Model file for the job. Use its own axes, mm. Face numbers are marked on the shaded views. A direction names the side the tool comes from. Give positions to 0.01 mm unless a question says otherwise; leave off trailing zeros. Answer in a Markdown table with one row per item.
```python
from build123d import *

# Parameters (mm, degrees)
SKETCH1_R                = 34.544
BOSS_EXTRUDE1_DEPTH      = 7.62
SKETCH2_R                = 28.1686
CUT_EXTRUDE1_DEPTH       = 3.048
CUT_EXTRUDE2_START       = -1.778
SKETCH3_R                = 28.1686
SKETCH3_R_2              = 4.3688
CUT_EXTRUDE2_DEPTH       = 1.778
CUT_EXTRUDE3_DEPTH       = 50.200658898
FILLET1_R                = 1.6002
CIRPATTERN1_COUNT        = 5
FILLET1_OF_CIRPATTERN1_R = 1.6002
SKETCH5_R                = 17.4625
SKETCH5_R_2              = 10.7061
BOSS_EXTRUDE2_DEPTH      = 1.778
BOSS_EXTRUDE4_START      = 1.6002
SKETCH6_R                = 17.4625
SKETCH6_R_2              = 16.4211
BOSS_EXTRUDE4_DEPTH      = 1.6002
SKETCH7_R                = 3.175
CUT_EXTRUDE4_DEPTH       = 50.066068275
SKETCH8_R                = 1.4224
CUT_EXTRUDE5_DEPTH       = 50.066068275
CIRPATTERN2_COUNT        = 5
BOSS_EXTRUDE5_DEPTH      = 0.0254
BOSS_EXTRUDE5_DEPTH_BACK = 7.6454
SKETCH9_R                = 34.5567
SKETCH9_R_2              = 30.4165


with BuildPart() as part:
    # Sketch1 → Boss-Extrude1 (new body)
    with BuildSketch(Plane(origin=(0, 0, 0), x_dir=(0, 0, -1), z_dir=(1, 0, 0))):
        with Locations(Location((0, 0, 0), (0, 0, 180))):
            Circle(SKETCH1_R)
    extrude(amount=BOSS_EXTRUDE1_DEPTH)

    # Sketch2 → Cut-Extrude1 (cut)
    with BuildSketch(Plane(origin=(7.62, 0, 0), x_dir=(0, 0, -1), z_dir=(1, 0, 0))):
        Circle(SKETCH2_R)
    extrude(amount=-CUT_EXTRUDE1_DEPTH, mode=Mode.SUBTRACT)

    # Sketch3 → Cut-Extrude2 (cut)
    with BuildSketch(Plane.ZY.offset(CUT_EXTRUDE2_START)):
        with Locations(Location((0, 0, 0), (0, 0, 180))):
            Circle(SKETCH3_R)
        Circle(SKETCH3_R_2, mode=Mode.SUBTRACT)
    extrude(amount=CUT_EXTRUDE2_DEPTH, mode=Mode.SUBTRACT)

    # Sketch4 → Cut-Extrude3 (cut, through all)
    with BuildSketch(Plane.ZY.offset(-1.778)):
        with BuildLine():
            Line((-2.54, 6.985), (2.54, 6.985))
            Line((2.54, 6.985), (9.114287493, 25.064290604))
            ThreePointArc((9.114287493, 25.064290604), (0, 26.67), (-9.114287493, 25.064290604))
            Line((-9.114287493, 25.064290604), (-2.54, 6.985))
        make_face()
    cut_extrude3 = extrude(amount=-CUT_EXTRUDE3_DEPTH, mode=Mode.SUBTRACT)

    # Fillet1
    fillet1_edges = [part.edges().sort_by_distance(p)[0] for p in [
        (3.175, 25.064290604, 9.114287493),
        (3.175, 6.985, 2.54),
        (3.175, 6.985, -2.54),
        (3.175, 25.064290604, -9.114287493),
    ]]
    fillet(fillet1_edges, radius=FILLET1_R)

    # CirPattern1: Cut-Extrude3 ×5 about axis
    cirpattern1_axis = Axis((0, 0, 0), (1, 0, 0))
    for i in range(1, CIRPATTERN1_COUNT):
        add(cut_extrude3.rotate(cirpattern1_axis, i * 360 / CIRPATTERN1_COUNT), mode=Mode.SUBTRACT)

    # Fillet1 of CirPattern1
    fillet1_of_cirpattern1_edges = [part.edges().sort_by_distance(p)[0] for p in [
        (3.175, -0.922910762, 26.654026632),
        (3.175, -0.257199846, 7.428032932),
        (3.175, 4.574167257, 5.858226601),
        (3.175, 16.41349426, 21.021087179),
        (3.175, -25.634680824, 7.358806903),
        (3.175, -7.143958247, 2.050776822),
        (3.175, -4.158009165, 6.160583153),
        (3.175, -14.920193278, 22.10603385),
        (3.175, -14.920193278, -22.10603385),
        (3.175, -4.158009165, -6.160583153),
        (3.175, -7.143958247, -2.050776822),
        (3.175, -25.634680824, -7.358806903),
        (3.175, 16.41349426, -21.021087179),
        (3.175, 4.574167257, -5.858226601),
        (3.175, -0.257199846, -7.428032932),
        (3.175, -0.922910762, -26.654026632),
    ]]
    fillet(fillet1_of_cirpattern1_edges, radius=FILLET1_OF_CIRPATTERN1_R)

    # Sketch5 → Boss-Extrude2 (add)
    with BuildSketch(Plane(origin=(4.572, 0, 0), x_dir=(0, 0, -1), z_dir=(1, 0, 0))):
        Circle(SKETCH5_R)
        Circle(SKETCH5_R_2, mode=Mode.SUBTRACT)
    extrude(amount=-BOSS_EXTRUDE2_DEPTH)

    # Sketch6 → Boss-Extrude4 (add)
    with BuildSketch(Plane(origin=(4.572, 0, 0), x_dir=(0, 0, -1), z_dir=(1, 0, 0)).offset(BOSS_EXTRUDE4_START)):
        Circle(SKETCH6_R)
        Circle(SKETCH6_R_2, mode=Mode.SUBTRACT)
    extrude(amount=-BOSS_EXTRUDE4_DEPTH)

    # Sketch7 → Cut-Extrude4 (cut, through all)
    with BuildSketch(Plane(origin=(4.572, 0, 0), x_dir=(0, 0, -1), z_dir=(1, 0, 0))):
        Circle(SKETCH7_R)
    extrude(amount=-CUT_EXTRUDE4_DEPTH, mode=Mode.SUBTRACT)

    # Sketch8 → Cut-Extrude5 (cut, through all)
    with BuildSketch(Plane(origin=(4.572, 0, 0), x_dir=(0, 0, -1), z_dir=(1, 0, 0))):
        with Locations((0, -6.35)):
            Circle(SKETCH8_R)
    cut_extrude5 = extrude(amount=-CUT_EXTRUDE5_DEPTH, mode=Mode.SUBTRACT)

    # CirPattern2: Cut-Extrude5 ×5 about axis
    cirpattern2_axis = Axis((0, 0, 0), (1, 0, 0))
    for i in range(1, CIRPATTERN2_COUNT):
        add(cut_extrude5.rotate(cirpattern2_axis, i * 360 / CIRPATTERN2_COUNT), mode=Mode.SUBTRACT)

    # Sketch9 → Boss-Extrude5 (add, two sides: drawn at the far end of the back side and taken through both)
    with BuildSketch(Plane(origin=(7.62, 0, 0), x_dir=(0, 0, -1), z_dir=(1, 0, 0)).offset(-BOSS_EXTRUDE5_DEPTH_BACK)):
        Circle(SKETCH9_R)
        Circle(SKETCH9_R_2, mode=Mode.SUBTRACT)
    extrude(amount=BOSS_EXTRUDE5_DEPTH + BOSS_EXTRUDE5_DEPTH_BACK)


solid = part.part
```
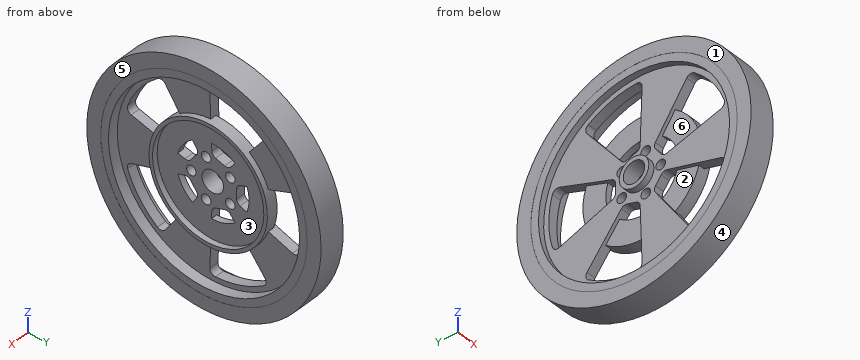
(1) Saw through at A-A, the plane y = -15. Count the separate pieces of the cut face and the enclosed holes in it, and give its area (3 significant figures).
Established:
| item | result |
|---|---|
| separate pieces | 3 |
| enclosed holes | 0 |
| area | 173 mm2 |
(2) Wall check: L1, parallel to Y at x = 0.4, z = 0 (3 decimals); L2, parallel to Y at x = 5.3, z = 0; L3, parallel to Z at x = 5.5, y = -10. Give the ranges that are in metal, low to high.
Established:
| item | result |
|---|---|
| L1 | y = -34.557 to -28.169, -4.369 to -3.175, 3.175 to 4.369, 28.169 to 34.557 |
| L2 | y = -34.56 to -28.17, -17.46 to -16.42, 16.42 to 17.46, 28.17 to 34.56 |
| L3 | z = -33.08 to -26.33, -14.32 to -13.03, 13.03 to 14.32, 26.33 to 33.08 |
(3) Flat gauge pins, fed straight in: P1, Ø10, axis at y = 0, z = 3.5, coming from the +X side; P2, Ø4.5, axis at y = 7, z = -12, coming from the -X side; P3, Ø2, axis at x = 1.5, y = 18, coming from the -Z side; P4, Ø2.5, axis at y = -6.35, z = 0, coming from the -X side. Where does each tip first touch, or does it go through?
Established:
| item | result |
|---|---|
| P1 | stops at x = 4.57 |
| P2 | stops at x = 1.78 |
| P3 | stops at z = -30.09 |
| P4 | passes through |
(4) Mould opens along Z. For the marked faces 4, 5 and 6 say: pulls with the +Z half, pulls with the -Z half, needs draft (parallel to the pull), parting line crosses it, or undercut.
Established:
| item | result |
|---|---|
| face 4 | parting line crosses it |
| face 5 | needs draft |
| face 6 | undercut |
(5) Which spindle directions (+Z, -Z, +X, -X, +Y, -Y) get a long thin tool onto all of the face, cutting with end or side? Do the marked faces 1, 2 and 3. Say none if no direction does.
Established:
| item | result |
|---|---|
| face 1 | +Z, -Z, -X, +Y, -Y |
| face 2 | -X |
| face 3 | +X |
